from build123d import *

# Parameters (mm, degrees)
ESQUISSE1_R                         = 27
ESQUISSE1_R_2                       = 24
ESQUISSE5_R                         = 17.3
ESQUISSE5_R_2                       = 14.3
BOSS_EXTRU_1_REACH                  = 108.661
BOSS_EXTRU_1_END_RADIUS             = 17.3
ESQUISSE8_R                         = 17.3
ESQUISSE8_R_2                       = 14.3
BOSS_EXTRU_1_DIRECTION_2_REACH      = 108.661
BOSS_EXTRU_1_DIRECTION_2_END_RADIUS = 27


with BuildPart() as part:
    # Balayage1: sweep along a path in Esquisse2
    with BuildLine(Plane(origin=(0, 0, 0), x_dir=(0, 0, -1), z_dir=(1, 0, 0))) as balayage1_path:
        Line((-35, 0), (35, 0))
    # Esquisse1 → Balayage1 (sweep)
    with BuildSketch(Plane.XY):
        Circle(ESQUISSE1_R)
        Circle(ESQUISSE1_R_2, mode=Mode.SUBTRACT)
    sweep(path=balayage1_path.line)



with BuildPart() as body_2:
    # Balayage2: sweep along a path in Esquisse6
    with BuildLine(Plane.XY) as balayage2_path:
        Line((110.918298302, -80.794444006), (110.918298302, -10.794444006))
    # Esquisse5 → Balayage2 (sweep)
    with BuildSketch(Plane(origin=(0, -45.794444006, 0), x_dir=(1, 0, 0), z_dir=(0, 1, 0))):
        with Locations((110.918298302, 0)):
            Circle(ESQUISSE5_R)
        with Locations((110.918298302, 0)):
            Circle(ESQUISSE5_R_2, mode=Mode.SUBTRACT)
    sweep(path=balayage2_path.line)


with BuildPart() as part_1:
    add(part.part)

    add(body_2.part)  # Boss.-Extru.1 merges body 2
    # Boss.-Extru.1: up to this cylinder (the profile starts outside it)
    boss_extru_1_end = Plane(origin=(110.918298302, -38.435657, 0), z_dir=(0, -1, 0)) * Cylinder(BOSS_EXTRU_1_END_RADIUS, 252.922, mode=Mode.PRIVATE)
    # Esquisse8 → Boss.-Extru.1 (add, up to the surface)
    with BuildSketch(Plane(origin=(55.459149151, -22.897222003, 0), x_dir=(0, 0, -1), z_dir=(0.9243191525163077, -0.381620366714795, 0)), mode=Mode.PRIVATE) as boss_extru_1_sk1:
        with Locations(Location((0, 0, 0), (0, 0, 90))):
            Circle(ESQUISSE8_R)
        with Locations(Location((0, 0, 0), (0, 0, 90))):
            Circle(ESQUISSE8_R_2, mode=Mode.SUBTRACT)
    boss_extru_1_tool1 = extrude(boss_extru_1_sk1.sketch, amount=BOSS_EXTRU_1_REACH, mode=Mode.PRIVATE) - boss_extru_1_end
    add(boss_extru_1_tool1.solids().sort_by_distance((49.04385, -38.435657, 0))[0])

    # Boss.-Extru.1 direction 2: up to this cylinder (the profile starts outside it)
    boss_extru_1_direction_2_end = Plane(origin=(0, 0, 0), z_dir=(0, 0, 1)) * Cylinder(BOSS_EXTRU_1_DIRECTION_2_END_RADIUS, 272.322, mode=Mode.PRIVATE)
    # Esquisse8 → Boss.-Extru.1 direction 2 (add, up to the surface)
    with BuildSketch(Plane(origin=(55.459149151, -22.897222003, 0), x_dir=(0, 0, -1), z_dir=(0.9243191525163077, -0.381620366714795, 0)), mode=Mode.PRIVATE) as boss_extru_1_direction_2_sk1:
        with Locations(Location((0, 0, 0), (0, 0, 90))):
            Circle(ESQUISSE8_R)
        with Locations(Location((0, 0, 0), (0, 0, 90))):
            Circle(ESQUISSE8_R_2, mode=Mode.SUBTRACT)
    boss_extru_1_direction_2_tool1 = extrude(boss_extru_1_direction_2_sk1.sketch, amount=-BOSS_EXTRU_1_DIRECTION_2_REACH, mode=Mode.PRIVATE) - boss_extru_1_direction_2_end
    add(boss_extru_1_direction_2_tool1.solids().sort_by_distance((49.04385, -38.435657, 0))[0])


solid = part_1.part
Work out the finished part from the listing and answer in its coordinate system (mm). A direction names the side the tool comes from. Coordinates: 2 decimals unless noted, no trailing zeros. Write each loop counter-clockwise with the first axis right and the second up, starting at its lowest first coordinate (ties: lowest second). Pieces come first, ordered by that corner, then holes. Notation, with made-up numbers: M 30.5,86 L 67.5,86 A18 cw 67.5,96 Z; hole C -34,-5 d8. An arc over 180 degrees is marked long. Use one line per item in the form item = value. Start each with the question number.
1. Straight lines are drawn through the part: probe 1 along Y at (x, z) = (0, -1); probe 2 along X at (y, z) = (1, 31.5); probe 3 along Z at (x, y) = (100, -40.5). For each, find the intervals that lie inside material, in ascending order. Write a range as from..to.
2. The part is cut by section C-C (y = 0). Give the number of separate pieces and of enclosed holes in the cut face, plus the area to 3 significant figures.
3. The part is cut by section A-A (x = 0). Give the vertices of the cut face in (y, z).
4. The part is cut by section B-B (z = 0). Give the vertices of the cut face in (x, y), plus the area to 3 significant figures.
5. Each of these flat-tipped pins is pushed along its axis until it touches: P1, Ø10, axis at x = 86.5, y = -49.5, coming from the -Z side; P2, Ø1.5, axis at x = 83, z = 7.5, coming from the +Y side; P3, Ø6, axis at y = -9, z = -24.5, coming from the +X side. Where does it stop, or does it pass through?
6. The mould has two halves that part along Y. Classify faces 3 (the face through (121.3, -80.794, -10.3)), 4 (the face through (121.3, -10.794, -10.3)), 5 (the face through (-23.977, -1.055, -0.49)): released by +Y, released by -Y, zero draft, split by the parting line, or undercut.
7. A tool of negligible diameter and unlimited length cuts with its end or side. For faces 1 (the face through (127.42, -45.3, -5.2)), 2 (the face through (-24.1, -1.9, 35)), from which of +Z, -Z, +X, -X, +Y, -Y can it reach the whole face along a straight path? Write none if from no direction.
8. The part is cut by section D-D (y = -62). Give the vertices of the cut face in (x, z), plus the area to 3 significant figures.
Evaluation:
q1.probe_1 = -27..-24, 24..27
q1.probe_2 = -26.98..-23.98, 23.98..26.98
q1.probe_3 = -17.28..-14.28, -13.42..-9.23, 9.23..13.42, 14.28..17.28
q2.separate_pieces = 2
q2.enclosed_holes = 1
q2.area = 633 mm^2
q3.outline = M -27,-35 L -24,-35 L -24,35 L -27,35 Z; M 24,-35 L 27,-35 L 27,35 L 24,35 Z
q4.outline = M 12.56,-23.9 L 93.62,-57.37 L 93.62,-80.79 L 96.62,-80.79 L 96.62,-10.79 L 93.62,-10.79 L 93.62,-19.94 L 25.76,8.08 A27 ccw long Z; M 125.22,-80.79 L 128.22,-80.79 L 128.22,-10.79 L 125.22,-10.79 Z; hole C 0,0 d48; hole M 15.71,-21.96 L 93.62,-54.12 L 93.62,-23.18 L 26.63,4.48 A27 cw Z
q4.area = 1,380 mm^2
q5.P1 = -15.47
q5.P2 = -16.92
q5.P3 = 26.32
q6.face_3 = released by -Y
q6.face_4 = released by +Y
q6.face_5 = undercut
q7.face_1 = none
q7.face_2 = +Z, +X, -X, +Y, -Y
q8.outline = C 110.92,0 d34.6; hole C 110.92,0 d28.6
q8.area = 298 mm^2
